The model under review builds one solid part; all positions refer to its coordinate system, in mm. A direction names the side the tool comes from. Coordinates: 2 decimals unless noted, no trailing zeros. Loops run counter-clockwise (first coordinate to the right, second up) from the corner with the lowest first, then second, coordinate; pieces in that order, holes last. Notation, with made-up numbers: M 56,-23.75 L 79,-23.75 A18 ccw 79,-18.75 Z; hole C 13.5,81.25 d10. An arc over 180 degrees is marked long. Write item = value, one per line. Start each with the question number.
Q1. We need section D-D on z = -2.5. Give the boundary of the cut face in (x, y), and give its area (3 significant figures).
Q2. Mouldability with a two-part tool opening along Y and no side actions: class faces 1 (the face through (65.02, 0.88, 20.07)), 2 (the face through (-85, 0, -15)), 3 (the face through (-114.993, -0.66, 12.325)), 4 (the face through (85, 0, 15)) as released by +Y, released by -Y, zero draft, split by the parting line, or undercut.
Q3. We need section B-B on y = 0. Give the boundary of the cut face in (x, z), and give its area (3 significant figures).
Q4. Clearance check with flat-ended pins moving along their axes: pin 1 Ø4 at (y, z) = (9.5, 13.5) entering from +X; pin 2 Ø3 at (y, z) = (-23.5, 6) entering from -X; pin 3 Ø3 at (y, z) = (-2.5, 20) entering from +X. State where each tip first meets the part, or that it passes through.
Q5. We need section C-C on x = -25.5. Give the boundary of the cut face in (y, z), and give its area (3 significant figures).
Q6. Wall thickness on probe 1 along Z at (x, y) = (-17, -20.5); probe 2 along Y at (x, z) = (85, 21.5); probe 3 along Z at (x, y) = (85.5, -14): over which ranges is each line inside the solid? List them lowest first.
Q7. We need section A-A on z = 21. Give the boundary of the cut face in (x, y).
Q8. For faces 5 (the face through (2, 0, 25)), 6 (the face through (-105.98, -0.92, -7.4)), list the 3-axis set-ups (+Z, -Z, +X, -X, +Y, -Y) from which the entire face can be reached by the end or side of a thin tool; tool diameter is ignored.
from build123d import *

# Parameters (mm, degrees)
SALIENTE_EXTRUIR1_DEPTH = 25
CROQUIS3_R              = 21
SALIENTE_EXTRUIR2_DEPTH = 15
CROQUIS4_R              = 20
CORTAR_EXTRUIR1_DEPTH   = 10


with BuildPart() as part:
    # Croquis2 → Saliente-Extruir1 (new body)
    with BuildSketch(Plane.XY):
        with BuildLine():
            Line((-85, 30), (85, 30))
            ThreePointArc((85, 30), (115, 0), (85, -30))
            Line((85, -30), (-85, -30))
            ThreePointArc((-85, -30), (-115, 0), (-85, 30))
        make_face()
    extrude(amount=SALIENTE_EXTRUIR1_DEPTH)

    # Croquis3 → Saliente-Extruir2 (add)
    with BuildSketch(Plane(origin=(0, 0, 0), x_dir=(-1, 0, 0), z_dir=(0, 0, -1))):
        with Locations(Location((85, 0, 0), (0, 0, 180))):
            Circle(CROQUIS3_R)
    extrude(amount=SALIENTE_EXTRUIR2_DEPTH)

    # Croquis4 → Cortar-Extruir1 (cut)
    with BuildSketch(Plane.XY.offset(25)):
        with Locations((85, 0)):
            Circle(CROQUIS4_R)
    extrude(amount=-CORTAR_EXTRUIR1_DEPTH, mode=Mode.SUBTRACT)


solid = part.part
Returned:
q1.outline = C -85,0 d42
q1.area = 1,390 mm^2
q2.face_1 = undercut
q2.face_2 = zero draft
q2.face_3 = split by the parting line
q2.face_4 = undercut
q3.outline = M -115,0 L -106,0 L -106,-15 L -64,-15 L -64,0 L 115,0 L 115,25 L 105,25 L 105,15 L 65,15 L 65,25 L -115,25 Z
q3.area = 5,980 mm^2
q4.pin_1 = 114.05
q4.pin_2 = -105.4
q4.pin_3 = 114.98
q5.outline = M -30,0 L 30,0 L 30,25 L -30,25 Z
q5.area = 1,500 mm^2
q6.probe_1 = 0 to 25
q6.probe_2 = -30 to -20, 20 to 30
q6.probe_3 = 0 to 15
q7.outline = M -85,-30 L 85,-30 A30 ccw 85,30 L -85,30 A30 ccw Z; hole C 85,0 d40
q8.face_5 = +Z, +X, -X, +Y, -Y
q8.face_6 = -Z
